Check sheet for the modelled part. Datum: model origin and axes. Units: mm. Face numbers are marked on the shaded views. A direction names the side the tool comes from. Round coordinates to 2 decimals unless told otherwise and drop trailing zeros. Order: outer loops, then holes, each group sorted by start corner. A loop starts at its lowest first (then second) coordinate and runs counter-clockwise, first axis right, second up.
Q1. Cross-section at D-D on y = -21.25. Record the cut outline in (x, z).
Q2. Scan lines: probe 1 along Z at (x, y) = (51.5, -10.25); probe 2 along X at (y, z) = (-9.5, -73); probe 3 along X at (y, z) = (0, -32.5). Record each from-to range of solid material in increasing order.
Q3. Cross-section at C-C on z = -62.5. Record the cut outline in (x, y), then the cut area to 3 significant figures.
Q4. Mould release check, pull along Z, two halves, no side actions. Record for the marked faces 1, 2, 3 and 4: +Z half, -Z half, draft (parallel to the pull), parting line (faces both ways), or undercut.
Q5. Depth check by flat-ended pin: P1, Ø5, axis at x = 15.82, y = -9.04, coming from the -Z side; P2, Ø5, axis at y = 1.5, z = -65, coming from the -X side; P3, Ø9, axis at y = -6, z = -36, coming from the -X side. Enter the tip coordinate at first touch or a pass-through.
Q6. Cross-section at B-B on x = 17.5. Record the cut outline in (y, z), then the cut area to 3 significant figures.
Q7. Cross-section at A-A on x = 73. Record the cut outline in (y, z), then the cut area to 3 significant figures.
Q8. Set-up check for the marked faces 5 and 6: record each of +Z, -Z, +X, -X, +Y, -Y from which the full face is reachable in a straight line by a thin tool's end or side.
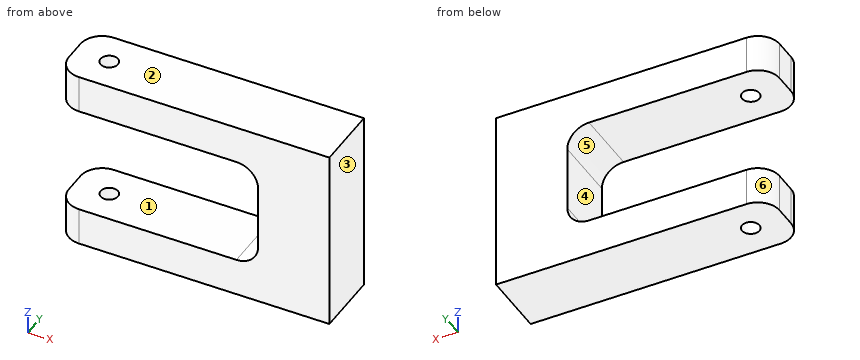
from build123d import *

# Parameters (mm, degrees)
EXTRUDE_START       = 7.5
EXTRUDE_1_DEPTH     = 85
SKETCH_3_W          = 94.594294475
SKETCH_3_H          = 50
CUT_EXTRUDE_1_DEPTH = 43.5
SKETCH_4_R          = 4
CUT_EXTRUDE_2_DEPTH = 100
FILLET_1_R          = 10


with BuildPart() as part:
    # Эскиз1 → Вытянуть1 (new body)
    with BuildSketch(Plane.XY.offset(EXTRUDE_START)):
        with BuildLine():
            Line((-0.114856082, -4.041900761), (-0.114856082, -14.041900761))
            ThreePointArc((-0.114856082, -14.041900761), (2.814076106, -21.112968573), (9.885143918, -24.041900761))
            Line((9.885143918, -24.041900761), (125.131658012, -24.041900761))
            Line((125.131658012, -24.041900761), (125.131658012, 5.958099239))
            Line((125.131658012, 5.958099239), (9.885143918, 5.958099239))
            ThreePointArc((9.885143918, 5.958099239), (2.814076106, 3.02916705), (-0.114856082, -4.041900761))
        make_face()
    extrude(amount=-EXTRUDE_1_DEPTH)

    # Эскиз3 → Вырез-Вытянуть1 (cut, symmetric)
    with BuildSketch(Plane(origin=(0, 0, 0), x_dir=(1, 0, 0), z_dir=(0, 1, 0))):
        with Locations((45.031047777, 35)):
            Rectangle(SKETCH_3_W, SKETCH_3_H)
    extrude(amount=CUT_EXTRUDE_1_DEPTH, both=True, mode=Mode.SUBTRACT)

    # Эскиз4 → Вырез-Вытянуть2 (cut, symmetric)
    with BuildSketch(Plane.XY):
        with Locations((15.823953055, -9.041900761)):
            Circle(SKETCH_4_R)
    extrude(amount=CUT_EXTRUDE_2_DEPTH, both=True, mode=Mode.SUBTRACT)

    # Скругление1
    fillet_1_edges = [part.edges().sort_by_distance(p)[0] for p in [
        (92.328195015, -9.041900761, -60),
        (92.328195015, -9.041900761, -10),
    ]]
    fillet(fillet_1_edges, radius=FILLET_1_R)


solid = part.part
Results found:
1. outline: (2.95, -77.5) - (125.13, -77.5) - (125.13, 7.5) - (2.95, 7.5) - (2.95, -10) - (82.33, -10) arc R10 cw to (92.33, -20) - (92.33, -50) arc R10 cw to (82.33, -60) - (2.95, -60) - close
2. probe 1: z = -77.5 to -60, -10 to 7.5
2. probe 2: x = -0.11 to 11.85, 19.8 to 125.13
2. probe 3: x = 92.33 to 125.13
3. outline: (-0.11, -14.04) arc R10 ccw to (9.89, -24.04) - (125.13, -24.04) - (125.13, 5.96) - (9.89, 5.96) arc R10 ccw to (-0.11, -4.04) - close; hole circle Ø8 at (15.82, -9.04)
3. area: 3,660 mm2
4. face 1: undercut
4. face 2: +Z half
4. face 3: draft
4. face 4: undercut
5. P1: passes through
5. P2: stops at x = 0.36
5. P3: stops at x = 92.33
6. outline: (-24.04, -77.5) - (-12.67, -77.5) - (-12.67, -60) - (-24.04, -60) - close; (-24.04, -10) - (-12.67, -10) - (-12.67, 7.5) - (-24.04, 7.5) - close; (-5.41, -77.5) - (5.96, -77.5) - (5.96, -60) - (-5.41, -60) - close; (-5.41, -10) - (5.96, -10) - (5.96, 7.5) - (-5.41, 7.5) - close
6. area: 796 mm2
7. outline: (-24.04, -77.5) - (5.96, -77.5) - (5.96, -60) - (-24.04, -60) - close; (-24.04, -10) - (5.96, -10) - (5.96, 7.5) - (-24.04, 7.5) - close
7. area: 1,050 mm2
8. face 5: -X, +Y, -Y
8. face 6: +Z, -Z, -X, +Y
